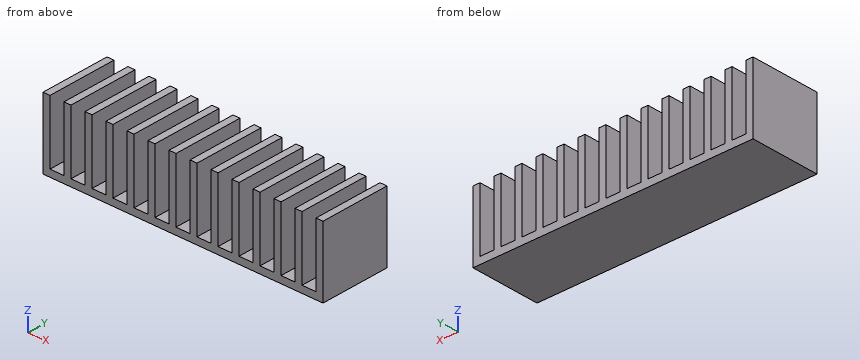
from build123d import *

# Parameters (mm, degrees)
F0_W     = 5
F0_H     = 50
F0_W_2   = 10
F1_DEPTH = 5
F2_DEPTH = 50


with BuildPart() as f1:
    # F0 (on Top) → F1 (new body)
    with BuildSketch(Plane.XY):
        with Locations((62.572898, -0.562236)):
            Rectangle(F0_W, F0_H)
        with Locations((40.072898, -0.562236)):
            Rectangle(F0_W_2, F0_H)
        with Locations((32.572898, -0.562236)):
            Rectangle(F0_W, F0_H)
        with Locations((-57.427102, -0.562236)):
            Rectangle(F0_W, F0_H)
        with Locations((2.572898, -0.562236)):
            Rectangle(F0_W, F0_H)
        with Locations((-94.927102, -0.562236)):
            Rectangle(F0_W_2, F0_H)
        with Locations((85.072898, -0.562236)):
            Rectangle(F0_W_2, F0_H)
        with Locations((77.572898, -0.562236)):
            Rectangle(F0_W, F0_H)
        with Locations((-4.927102, -0.562236)):
            Rectangle(F0_W_2, F0_H)
        with Locations((-34.927102, -0.562236)):
            Rectangle(F0_W_2, F0_H)
        with Locations((92.572898, -0.562236)):
            Rectangle(F0_W, F0_H)
        with Locations((-72.427102, -0.562236)):
            Rectangle(F0_W, F0_H)
        with Locations((70.072898, -0.562236)):
            Rectangle(F0_W_2, F0_H)
        with Locations((-42.427102, -0.562236)):
            Rectangle(F0_W, F0_H)
        with Locations((-49.927102, -0.562236)):
            Rectangle(F0_W_2, F0_H)
        with Locations((25.072898, -0.562236)):
            Rectangle(F0_W_2, F0_H)
        with Locations((10.072898, -0.562236)):
            Rectangle(F0_W_2, F0_H)
        with Locations((-64.927102, -0.562236)):
            Rectangle(F0_W_2, F0_H)
        with Locations((47.572898, -0.562236)):
            Rectangle(F0_W, F0_H)
        with Locations((-79.927102, -0.562236)):
            Rectangle(F0_W_2, F0_H)
        with Locations((-27.427102, -0.562236)):
            Rectangle(F0_W, F0_H)
        with Locations((-102.427102, -0.562236)):
            Rectangle(F0_W, F0_H)
        with Locations((-12.427102, -0.562236)):
            Rectangle(F0_W, F0_H)
        with Locations((-19.927102, -0.562236)):
            Rectangle(F0_W_2, F0_H)
        with Locations((-87.427102, -0.562236)):
            Rectangle(F0_W, F0_H)
        with Locations((55.072898, -0.562236)):
            Rectangle(F0_W_2, F0_H)
        with Locations((17.572898, -0.562236)):
            Rectangle(F0_W, F0_H)
    extrude(amount=F1_DEPTH)

    # F0 (on Top) → F2 (join)
    with BuildSketch(Plane.XY):
        with Locations((-102.427102, -0.562236)):
            Rectangle(F0_W, F0_H)
        with Locations((-87.427102, -0.562236)):
            Rectangle(F0_W, F0_H)
        with Locations((-72.427102, -0.562236)):
            Rectangle(F0_W, F0_H)
        with Locations((-57.427102, -0.562236)):
            Rectangle(F0_W, F0_H)
        with Locations((-42.427102, -0.562236)):
            Rectangle(F0_W, F0_H)
        with Locations((-27.427102, -0.562236)):
            Rectangle(F0_W, F0_H)
        with Locations((-12.427102, -0.562236)):
            Rectangle(F0_W, F0_H)
        with Locations((2.572898, -0.562236)):
            Rectangle(F0_W, F0_H)
        with Locations((17.572898, -0.562236)):
            Rectangle(F0_W, F0_H)
        with Locations((32.572898, -0.562236)):
            Rectangle(F0_W, F0_H)
        with Locations((47.572898, -0.562236)):
            Rectangle(F0_W, F0_H)
        with Locations((62.572898, -0.562236)):
            Rectangle(F0_W, F0_H)
        with Locations((77.572898, -0.562236)):
            Rectangle(F0_W, F0_H)
        with Locations((92.572898, -0.562236)):
            Rectangle(F0_W, F0_H)
    extrude(amount=F2_DEPTH)


solid = f1.part
Could you check a few things on this model? Use its own coordinates, in mm. Give positions to 0.01 mm unless a question says otherwise; leave off trailing zeros. Order: outer loops, then holes, each group sorted by start corner. A loop starts at its lowest first (then second) coordinate and runs counter-clockwise, first axis right, second up.
1. Suppose I cut it at B-B (x = 28). List the corners of the cut face in (y, z) for me, plus the area to 3 significant figures.
2. I need wall thicknesses on L1, parallel to Z at x = 15, y = 8. Which ranges of the line are inside material? Lowest first, please.
3. Will this pin go through, and if not, where does the flat tip stop? P1, Ø2, axis at x = -62.5, y = 0.5, coming from the +Z side.
4. Suppose I cut it at A-A (z = 21). Give the number of separate pieces and of enclosed holes in the cut face, plus the area to 3 significant figures.
Solved:
1. outline: (-25.56, 0) - (24.44, 0) - (24.44, 5) - (-25.56, 5) - close
1. area: 250 mm2
2. L1: z = 0 to 5
3. P1: stops at z = 5
4. separate pieces: 14
4. enclosed holes: 0
4. area: 3,500 mm2
